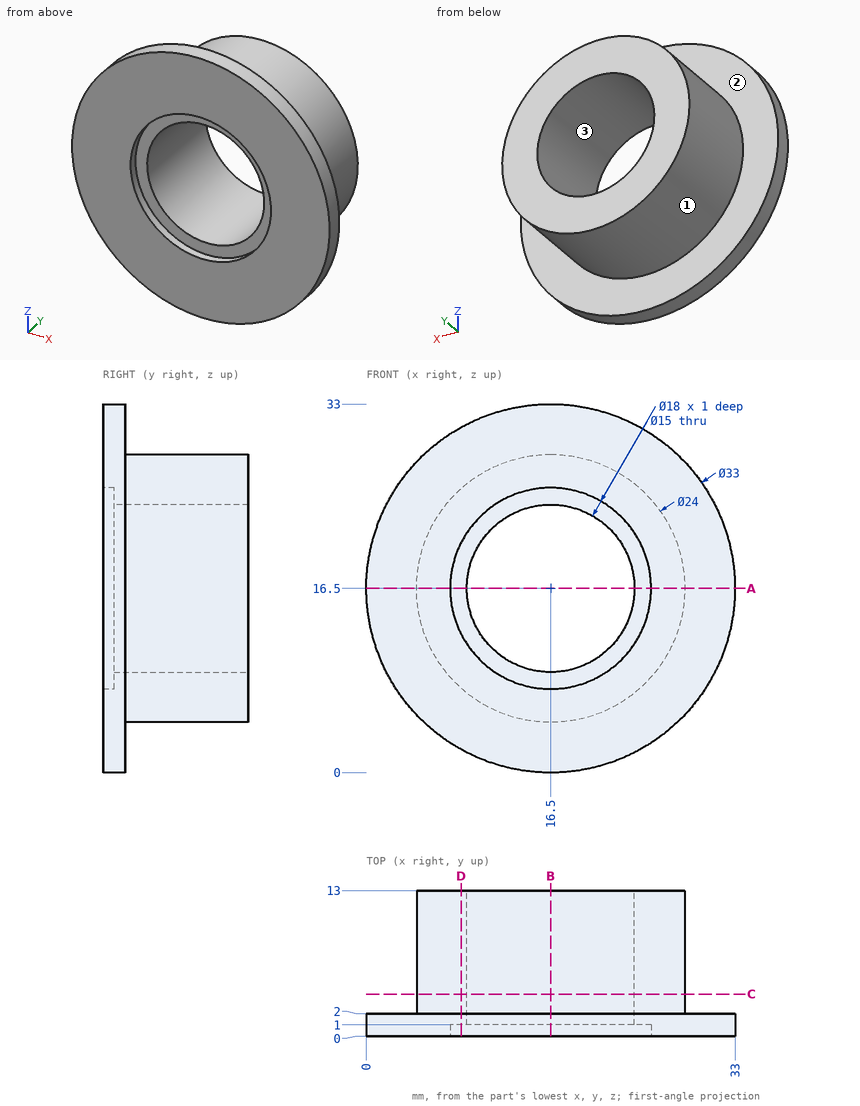
The drawing under review shows one solid part. Ordinate dimensions are in mm from its lowest x, y, z. Coordinates: 2 decimals unless noted, no trailing zeros. Write each loop counter-clockwise with the first axis right and the second up, starting at its lowest first coordinate (ties: lowest second). Pieces come first, ordered by that corner, then holes.
1) Insertion check: pin 1 (4 mm diameter, centred on y = 10.5, z = 24.5, fed in from -X); pin 2 (6 mm diameter, centred on y = 9.5, z = 6, fed in from -X); pin 3 (11 mm diameter, centred on x = 16.5, z = 16.5, fed in from +Y); pin 4 (17 mm diameter, centred on x = 16.5, z = 16.5, fed in from -Y). Each pin has a flat end and moves straight along its axis. Give the tip position at first contact, or say it passes through.
2) Mouldability with a two-part tool opening along Z and no side actions: class the marked faces 1, 2 and 3 as +Z half, -Z half, draft (parallel to the pull), parting line (faces both ways), or undercut.
3) Add section B-B (x = 16.5). Write out the cut boundary in (y, z).
4) Add section D-D (x = 8.5). Write out the cut boundary in (y, z).
5) To check wall thickness, follow L1, parallel to X at y = 0.45, z = 16.5; L2, parallel to X at y = 5.5, z = 16.5; L3, parallel to Y at x = 8, z = 16. State the ranges of each line that lie inside material, in increasing order.
6) Add section A-A (z = 16.5). Write out the cut boundary in (x, y), plus the area to 3 significant figures.
7) Add section C-C (y = 3.75). Write out the cut boundary in (x, z).
Check result:
1. pin 1: stops at x = 6.11
1. pin 2: stops at x = 7.13
1. pin 3: passes through
1. pin 4: stops at y = 1
2. face 1: parting line
2. face 2: draft
2. face 3: undercut
3. outline: (0, 0) - (2, 0) - (2, 4.5) - (13, 4.5) - (13, 9) - (1, 9) - (1, 7.5) - (0, 7.5) - close; (0, 25.5) - (1, 25.5) - (1, 24) - (13, 24) - (13, 28.5) - (2, 28.5) - (2, 33) - (0, 33) - close
4. outline: (0, 2.07) - (2, 2.07) - (2, 7.56) - (13, 7.56) - (13, 25.44) - (2, 25.44) - (2, 30.93) - (0, 30.93) - (0, 20.62) - (1, 20.62) - (1, 12.38) - (0, 12.38) - close
5. L1: x = 0 to 7.5, 25.5 to 33
5. L2: x = 4.5 to 9, 24 to 28.5
5. L3: y = 1 to 13
6. outline: (0, 0) - (7.5, 0) - (7.5, 1) - (9, 1) - (9, 13) - (4.5, 13) - (4.5, 2) - (0, 2) - close; (24, 1) - (25.5, 1) - (25.5, 0) - (33, 0) - (33, 2) - (28.5, 2) - (28.5, 13) - (24, 13) - close
6. area: 132 mm2
7. outline: circle Ø24 at (16.5, 16.5); hole circle Ø15 at (16.5, 16.5)
